Can you work these out from the model? Positions are in its coordinate system, mm. Face numbers are marked on the shaded views. A direction names the side the tool comes from. Coordinates: 2 decimals unless noted, no trailing zeros. Order: outer loops, then holes, each group sorted by start corner. A loop starts at its lowest first (then second) coordinate and runs counter-clockwise, first axis right, second up. Notation, with made-up numbers: M -14,-32 L 25,-32 A29 ccw 25,-7 Z; hole C -14.75,-3 d11. An arc over 180 degrees is marked long. Answer as a JSON object with one key per item and string values.
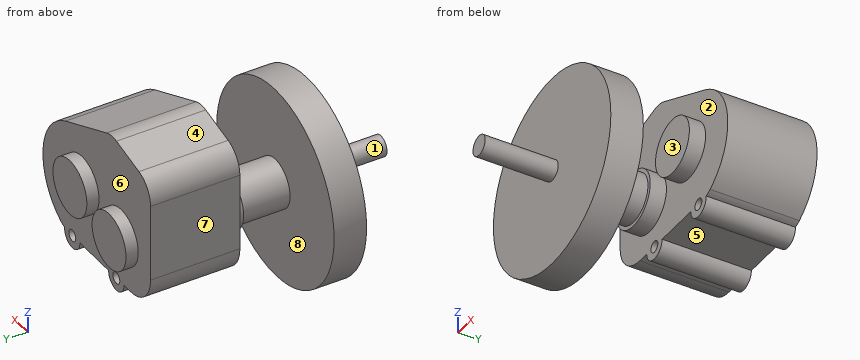
from build123d import *

# Parameters (mm, degrees)
F1_DEPTH      = 69.85
F2_R          = 22
F3_DEPTH      = 79.375
F3_DEPTH_BACK = 12.7
F4_R          = 10
F5_DEPTH      = 69.85
F6_R          = 4.5
F7_DEPTH      = 82.551
F8_R          = 19.05
F9_DEPTH      = 38.1
F10_R         = 7.9375
F11_DEPTH     = 82.55
F12_R         = 76.2
F13_DEPTH     = 25.4


# Not quite as in the source:
# - a length typed as a fraction of an inch, garbled in the dataset ("3 / 203.2 mm" for 3/8 in), is restored


with BuildPart() as f1:
    # F0 (on Front) → F1 (new body)
    with BuildSketch(Plane.XZ):
        with BuildLine():
            ThreePointArc((-32.4406404125, 46.3256966582), (-43.3540366721, 39.2310908433), (-47.5899279118, 26.9228466552))
            Line((-47.5899279118, 26.9228466552), (-47.5899279118, -33.6616252167))
            ThreePointArc((-47.5899279118, -33.6616252167), (-40.1504401539, -51.6221374588), (-22.1899279118, -59.0616252167))
            Line((-22.1899279118, -59.0616252167), (58.6284401518, -59.0616252167))
            ThreePointArc((58.6284401518, -59.0616252167), (64.1154300354, -58.2942262372), (69.1813488754, -56.0509194183))
            ThreePointArc((69.1813488754, -56.0509194183), (91.9687648373, -11.1091837062), (62.6034215093, 29.8383747833))
            Line((62.6034215093, 29.8383747833), (9.3969636816, 52.592505372))
            ThreePointArc((9.3969636816, 52.592505372), (3.1225085413, 54.1402430548), (-3.3179311218, 53.6063739808))
            Line((-3.3179311218, 53.6063739808), (-32.4406404125, 46.3256966582))
        make_face()
    extrude(amount=F1_DEPTH)

    # F2 (on face) → F3 (join, two sides)
    with BuildSketch(Plane.XZ.offset(69.85)) as f3_sk:
        with Locations((-9.4899279118, -20.9616252167)):
            Circle(F2_R)
        with Locations((41.3100720882, -8.2616252167)):
            Circle(F2_R)
    extrude(amount=-F3_DEPTH)
    extrude(f3_sk.sketch, amount=F3_DEPTH_BACK)

    # F4 (on face) → F5 (join, through all)
    with BuildSketch(Plane(origin=(0, 0, 0), x_dir=(-1, 0, 0), z_dir=(0, 1, 0))):
        with Locations((-54.0100720882, -59.0616252167)):
            Circle(F4_R)
        with Locations((3.1399279118, -59.0616252167)):
            Circle(F4_R)
    extrude(amount=-F5_DEPTH)

    # F6 (on face) → F7 (cut, through all)
    with BuildSketch(Plane(origin=(0, 0, 0), x_dir=(-1, 0, 0), z_dir=(0, 1, 0))):
        with Locations((-54.0100720882, -59.0616252167)):
            Circle(F6_R)
        with Locations((3.1399279118, -59.0616252167)):
            Circle(F6_R)
    extrude(amount=-F7_DEPTH, mode=Mode.SUBTRACT)

    # F8 (on face) → F9 (join)
    with BuildSketch(Plane.XZ.offset(82.55)):
        with Locations((-9.4899279118, -20.9616252167)):
            Circle(F8_R)
    extrude(amount=F9_DEPTH)

    # F10 (on face) → F11 (join)
    with BuildSketch(Plane.XZ.offset(120.65)):
        with Locations((-9.4899279118, -20.9616252167)):
            Circle(F10_R)
    extrude(amount=F11_DEPTH)

    # F12 (on face) → F13 (join)
    with BuildSketch(Plane.XZ.offset(120.65)):
        with Locations((-9.4899279118, -20.9616252167)):
            Circle(F12_R)
    extrude(amount=F13_DEPTH)


solid = f1.part
Item 1: I want a section at A-A, the plane y = -26. Write out the boundary of the cut face in (x, z), plus the area to 3 significant figures.
Answers follow:
{"outline": "M -47.59,-33.66 A25.4 ccw -22.19,-59.06 L -13.14,-59.06 A10 ccw 6.86,-59.06 L 44.01,-59.06 A10 ccw long 63.98,-58.33 A20 ccw 69.18,-56.05 A48.54 ccw 62.6,29.84 L 9.4,52.59 A20 ccw -3.32,53.61 L -32.44,46.33 A20 ccw -47.59,26.92 Z; hole C -3.14,-59.06 d9; hole C 54.01,-59.06 d9", "area": "13,400 mm^2"}
Item 2: I want a section at C-C, the plane z = -87. Write out the boundary of the cut face in (x, y), plus the area to 3 significant figures.
Answers follow:
{"outline": "M -47.51,-146.05 L 28.53,-146.05 L 28.53,-120.65 L -47.51,-120.65 Z", "area": "1,930 mm^2"}
Item 3: I'm going to push flat-ended pins straight in: pin 1 (6 mm diameter, centred on y = -80, z = -44, fed in from +X); pin 2 (4 mm diameter, centred on x = -19.5, z = -48, fed in from +Y); pin 3 (4 mm diameter, centred on x = -53, z = -14, fed in from +Y). Where does each tip first touch, or does it pass through?
Answers follow:
{"pin 1": "stops at x = -0.41", "pin 2": "stops at y = 0", "pin 3": "stops at y = -120.65"}
Item 4: I want a section at B-B, the plane y = -78. Write out the boundary of the cut face in (x, z).
Answers follow:
{"outline": "C -9.49,-20.96 d44; C 41.31,-8.26 d44"}
Item 5: I want a section at D-D, the plane x = 72. Write out the boundary of the cut face in (y, z).
Answers follow:
{"outline": "M -69.85,-54.16 L 0,-54.16 L 0,24.53 L -69.85,24.53 Z"}
Item 6: Which directions (+Z, -Z, +X, -X, +Y, -Y) give clear straight access to the entire face, cutting with the end or side of a thin tool? Please do the marked faces 1, 2, 3, 4 and 5.
Answers follow:
{"face 1": "-Y", "face 2": "none", "face 3": "+Z, -Z, +X", "face 4": "+Z, -X, +Y", "face 5": "-Z, +Y"}
Item 7: Please list where these lines run through material, in increasing order: line 1 (Y direction, x = 27.5, z = -14) (3 decimals); line 2 (Y direction, x = 60, z = -39); line 3 (Y direction, x = -52.5, z = -74).
Answers follow:
{"line 1": "y = -146.05 to -120.65, -82.55 to 9.525", "line 2": "y = -146.05 to -120.65, -69.85 to 0", "line 3": "y = -146.05 to -120.65"}
Item 8: If we mould it in two halves opening along Y, with no side actions, what happens to the marked faces 6, 7 and 8? For each: pulls with the +Y half, pulls with the -Y half, needs draft (parallel to the pull), parting line crosses it, or undercut.
Answers follow:
{"face 6": "pulls with the +Y half", "face 7": "needs draft", "face 8": "undercut"}
